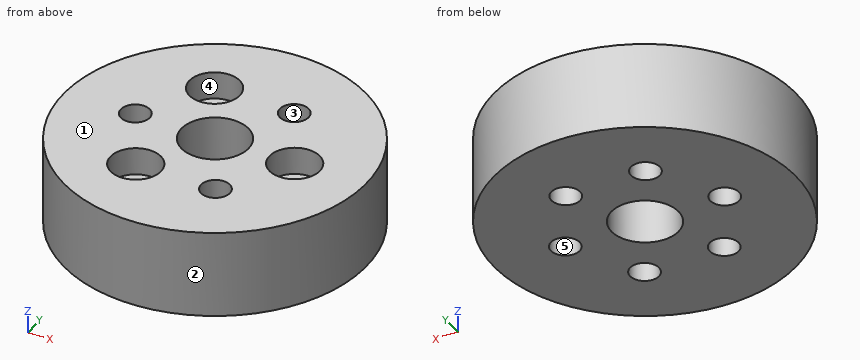
from build123d import *

# Parameters (mm, degrees)
SKETCH2_R           = 22.5
SKETCH2_R_2         = 2.15
BOSS_EXTRUDE1_DEPTH = 13
SKETCH3_R           = 3.75
CUT_EXTRUDE1_DEPTH  = 4.1
SKETCH5_R           = 5
CUT_EXTRUDE3_DEPTH  = 35.372954485


with BuildPart() as part:
    # Sketch2 → Boss-Extrude1 (new body)
    with BuildSketch(Plane.XY):
        with Locations(Location((0, 0, 0), (0, 0, 180))):
            Circle(SKETCH2_R)
        with Locations(Location((12, 0, 0), (0, 0, 180))):
            Circle(SKETCH2_R_2, mode=Mode.SUBTRACT)
        with Locations(Location((6, -10.392304845, 0), (0, 0, 180))):
            Circle(SKETCH2_R_2, mode=Mode.SUBTRACT)
        with Locations(Location((-6, -10.392304845, 0), (0, 0, 180))):
            Circle(SKETCH2_R_2, mode=Mode.SUBTRACT)
        with Locations(Location((-12, 0, 0), (0, 0, 180))):
            Circle(SKETCH2_R_2, mode=Mode.SUBTRACT)
        with Locations(Location((-6, 10.392304845, 0), (0, 0, 180))):
            Circle(SKETCH2_R_2, mode=Mode.SUBTRACT)
        with Locations(Location((6, 10.392304845, 0), (0, 0, 180))):
            Circle(SKETCH2_R_2, mode=Mode.SUBTRACT)
    extrude(amount=BOSS_EXTRUDE1_DEPTH)

    # Sketch3 → Cut-Extrude1 (cut)
    with BuildSketch(Plane.XY.offset(13)):
        with Locations((-6, 10.392304845)):
            Circle(SKETCH3_R)
        with Locations((-6, -10.392304845)):
            Circle(SKETCH3_R)
        with Locations((12, 0)):
            Circle(SKETCH3_R)
    extrude(amount=-CUT_EXTRUDE1_DEPTH, mode=Mode.SUBTRACT)

    # Sketch5 → Cut-Extrude3 (cut, through all)
    with BuildSketch(Plane.XY.offset(13)):
        Circle(SKETCH5_R)
    extrude(amount=-CUT_EXTRUDE3_DEPTH, mode=Mode.SUBTRACT)


solid = part.part
Geometry: final body of the model. Coordinates: model frame, mm. Face numbers are marked on the shaded views. A direction names the side the tool comes from. Coordinates: 2 decimals unless noted, no trailing zeros. Order: outer loops, then holes, each group sorted by start corner. A loop starts at its lowest first (then second) coordinate and runs counter-clockwise, first axis right, second up. Notation, with made-up numbers: M -5.75,-13 L 0.25,-13 A14 cw 0.25,-8 Z; hole C 70,72 d8. An arc over 180 degrees is marked long. One line per question, with ' | ' between items. Start each with the question number.
Item 1: Cut plane B-B, the plane y = 0. Return the cut outline in (x, z), then the cut area to 3 significant figures.
Item 2: Cut plane D-D, the plane x = -6. Return the cut outline in (y, z).
Item 3: Cut plane A-A, the plane x = 0. Return the cut outline in (y, z).
Item 4: Ray query, probe 1 along Y at (x, z) = (-6, 10.85); probe 2 along X at (y, z) = (10.5, 3); probe 3 along Y at (x, z) = (-6, 3.5). Return the intervals inside material, ascending. Write a range as [from, to].
Item 5: Draft query along X for the marked faces 1, 2 and 3. Return one class per face: released by +X, released by -X, zero draft, split by the parting line, or undercut.
Item 6: Pin query (flat end, axial travel): pin 1 Ø5.5 at (x, y) = (6, 10.39) entering from +Z; pin 2 Ø3 at (x, z) = (1, 5) entering from +Y; pin 3 Ø1.5 at (y, z) = (14, 6) entering from -X; pin 4 Ø4 at (x, y) = (-5, 9.5) entering from +Z. Return the tip coordinate at first contact, or that it passes through.
Item 7: Set-up query: the marked faces 4 and 5. Return all of +Z, -Z, +X, -X, +Y, -Y with unobstructed straight access to the full face (end or side cutting, diameter ignored); none if empty.
Item 8: Cut plane C-C, the plane z = 3. Return the cut outline in (x, y), then the cut area to 3 significant figures.
A:
1) outline: M -22.5,0 L -14.15,0 L -14.15,13 L -22.5,13 Z; M -9.85,0 L -5,0 L -5,13 L -9.85,13 Z; M 5,0 L 9.85,0 L 9.85,8.9 L 8.25,8.9 L 8.25,13 L 5,13 Z; M 14.15,0 L 22.5,0 L 22.5,13 L 15.75,13 L 15.75,8.9 L 14.15,8.9 Z | area: 330 mm2
2) outline: M -21.69,0 L -12.54,0 L -12.54,8.9 L -14.14,8.9 L -14.14,13 L -21.69,13 Z; M -8.24,0 L 8.24,0 L 8.24,8.9 L 6.64,8.9 L 6.64,13 L -6.64,13 L -6.64,8.9 L -8.24,8.9 Z; M 12.54,0 L 21.69,0 L 21.69,13 L 14.14,13 L 14.14,8.9 L 12.54,8.9 Z
3) outline: M -22.5,0 L -5,0 L -5,13 L -22.5,13 Z; M 5,0 L 22.5,0 L 22.5,13 L 5,13 Z
4) probe 1: y = [-21.69, -14.14], [-6.64, 6.64], [14.14, 21.69] | probe 2: x = [-19.9, -8.15], [-3.85, 3.85], [8.15, 19.9] | probe 3: y = [-21.69, -12.54], [-8.24, 8.24], [12.54, 21.69]
5) face 1: zero draft | face 2: split by the parting line | face 3: undercut
6) pin 1: stops at z = 13 | pin 2: stops at y = 22.5 | pin 3: stops at x = -18.18 | pin 4: stops at z = 8.9
7) face 4: +Z | face 5: +Z, -Z
8) outline: C 0,0 d45; hole C -12,0 d4.3; hole C -6,-10.39 d4.3; hole C -6,10.39 d4.3; hole C 0,0 d10; hole C 6,-10.39 d4.3; hole C 6,10.39 d4.3; hole C 12,0 d4.3 | area: 1,420 mm2
